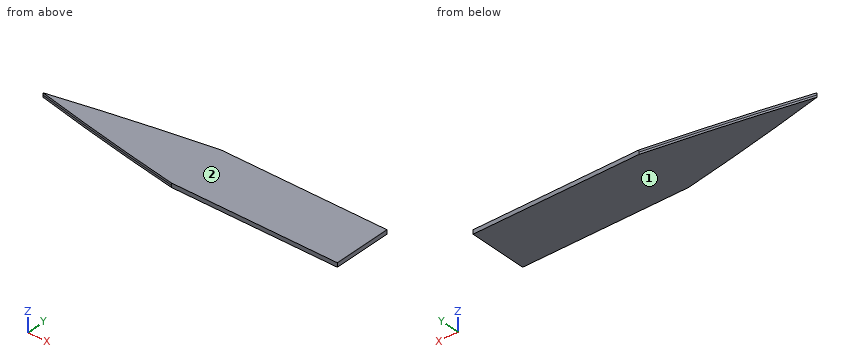
```python
from build123d import *

# Parameters (mm, degrees)
BOSS_EXTRUDE1_DEPTH      = 1.25
BOSS_EXTRUDE1_DEPTH_BACK = 1.25


with BuildPart() as part:
    # Sketch2 → Boss-Extrude1 (new body, two sides)
    with BuildSketch(Plane.XY) as boss_extrude1_sk:
        with BuildLine():
            Line((98.502891266, 17.588765104), (198.502891266, 17.588765104))
            Line((198.502891266, 17.588765104), (198.502891266, -17.588765104))
            Line((198.502891266, -17.588765104), (98.502891266, -17.588765104))
            add(Edge.make_bspline(
                [(6.253387475, 0), (52.148844411, -9.975392509), (98.502891266, -17.588765104)],
                knots=[0, 0, 0, 1, 1, 1], degree=2))
            add(Edge.make_bspline(
                [(6.253387475, 0), (52.148844411, 9.975392509), (98.502891266, 17.588765104)],
                knots=[0, 0, 0, 1, 1, 1], degree=2))
        make_face()
    extrude(amount=BOSS_EXTRUDE1_DEPTH)
    extrude(boss_extrude1_sk.sketch, amount=-BOSS_EXTRUDE1_DEPTH_BACK)


solid = part.part
```
Here's how the part is built. I have some questions about the finished solid (model axes, mm). Face numbers are marked on the shaded views. Give positions to 0.01 mm unless a question says otherwise; leave off trailing zeros. Answer as a JSON object with one key per item and string values. Group by question number.
Item 1: Please list where these lines run through material, in increasing order: probe 1 along Y at (x, z) = (54.5, 1); probe 2 along Y at (x, z) = (80.5, -0.1).
Item 2: For P1, Ø1, axis at x = 71, z = 1, coming from the -Y side, with a flat end and sliding along its axis, tell me the tip position at first contact or that it passes through.
Item 3: If we mould it in two halves opening along Z, with no side actions, what happens to the marked faces 1 and 2? For each: pulls with the +Z half, pulls with the -Z half, needs draft (parallel to the pull), parting line crosses it, or undercut.
Result set:
{
 "1": {"probe 1": "-9.81 to 9.81", "probe 2": "-14.54 to 14.54"},
 "2": {"P1": "y = -12.95"},
 "3": {"face 1": "pulls with the -Z half", "face 2": "pulls with the +Z half"}
}
